Verification items for the finished model (mm, model axes). Give positions to 0.01 mm unless a question says otherwise; leave off trailing zeros. Write each loop counter-clockwise with the first axis right and the second up, starting at its lowest first coordinate (ties: lowest second). Pieces come first, ordered by that corner, then holes. Notation, with made-up numbers: (78, 61.25) - (108, 61.25) arc R14 ccw to (108, 81.25) - close; hole circle Ø1 at (-1.75, 47.25). An arc over 180 degrees is marked (long way). Answer as a JSON object with one key per item and string values. Group by question number.
Item 1: Go/stop test with flat-tipped pins: pin 1 (4 mm diameter, centred on x = -16.5, z = -257, fed in from -Y); pin 2 (6 mm diameter, centred on y = 30, z = -389.5, fed in from +X); pin 3 (3 mm diameter, centred on x = -17.5, z = -315.5, fed in from -Y); pin 4 (3 mm diameter, centred on x = -4, y = 11, fed in from -Z). Record where each tip stops, or that it passes through.
Item 2: Sectioned sample at A-A, the plane z = -415. Record the boundary of the cut face in (x, y).
Item 3: Sectioned sample at B-B, the plane y = 17.5. Record the boundary of the cut face in (x, z), and give its area (3 significant figures).
Item 4: Scan lines: line 1 along Y through (x, z) = (-16.5, -194); line 2 along X through (y, z) = (3.5, -122); line 3 along X through (y, z) = (40.5, -39). Record each from-to range of solid material in increasing order. Write a range as [from, to].
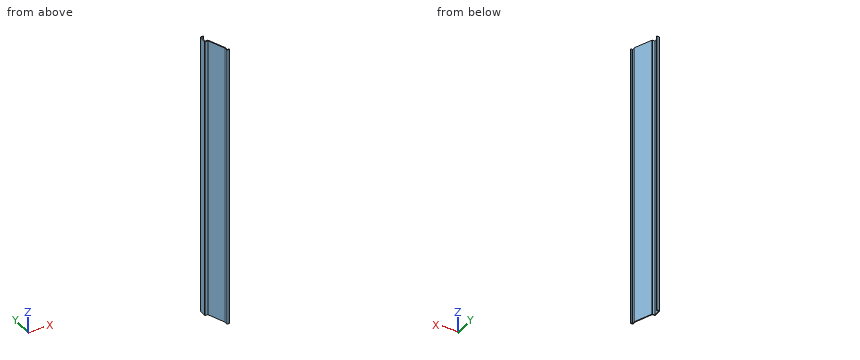
```python
from build123d import *

# Parameters (mm, degrees)
EXTRUDE_THIN1_DEPTH = 444.5
FILLET1_R           = 1.27


with BuildPart() as part:
    # Sketch1 → Extrude-Thin1 (new body)
    with BuildSketch(Plane.XY):
        Polygon((0, 0), (-3.96875, 0), (-3.96875, 5.55625), (-15.08125, 31.75), (-19.84375, 31.75), (-19.84375, 44.45), (-15.08125, 44.45), (-15.08125, 43.18), (-18.57375, 43.18), (-18.57375, 33.02), (-14.240475492, 33.02), (-2.69875, 5.814504197), (-2.69875, 1.27), (0, 1.27), align=None)
    extrude(amount=-EXTRUDE_THIN1_DEPTH)

    # Fillet1
    fillet1_edges = [part.edges().sort_by_distance(p)[0] for p in [
        (-14.240475492, 33.02, -222.25),
        (-2.69875, 5.814504197, -222.25),
        (-3.96875, 0, -222.25),
        (-19.84375, 31.75, -222.25),
        (-19.84375, 44.45, -222.25),
    ]]
    fillet(fillet1_edges, radius=FILLET1_R)


solid = part.part
```
Geometry check:
{
 "1": {"pin 1": "y = 30.38", "pin 2": "x = -11.69", "pin 3": "y = 31.75", "pin 4": "z = -444.5"},
 "2": {"outline": "(-19.84, 33.02) arc R1.27 ccw to (-18.57, 31.75) - (-15.08, 31.75) - (-3.97, 5.56) - (-3.97, 1.27) arc R1.27 ccw to (-2.7, 0) - (0, 0) - (0, 1.27) - (-2.7, 1.27) - (-2.7, 5.56) arc R1.27 ccw to (-2.8, 6.05) - (-13.91, 32.25) arc R1.27 ccw to (-15.08, 33.02) - (-18.57, 33.02) - (-18.57, 43.18) - (-15.08, 43.18) - (-15.08, 44.45) - (-18.57, 44.45) arc R1.27 ccw to (-19.84, 43.18) - close"},
 "3": {"outline": "(-9.04, -444.5) - (-7.66, -444.5) - (-7.66, 0) - (-9.04, 0) - close", "area": "613 mm^2"},
 "4": {"line 1": "[31.75, 33.02], [43.18, 44.45]", "line 2": "[-3.97, -2.7]", "line 3": "[-19.84, -18.57]"}
}
